from build123d import *

# Parameters (mm, degrees)
F0_W     = 21
F0_H     = 21
F1_DEPTH = 11
F3_DEPTH = 21.001
F5_DEPTH = 25
F6_W     = 0.76
F6_H     = 0.76
F7_DEPTH = 5.8


with BuildPart() as f1:
    # F0 (on Top) → F1 (new body)
    with BuildSketch(Plane.XY):
        with Locations((10.5, 10.5)):
            Rectangle(F0_W, F0_H)
    extrude(amount=F1_DEPTH)

    # F2 (on face) → F3 (cut, through all)
    with BuildSketch(Plane.XZ):
        Polygon((0, 11), (0, 0), (0.6, 11), align=None)
        Polygon((20.4, 11), (21, 0), (21, 11), align=None)
    extrude(amount=-F3_DEPTH, mode=Mode.SUBTRACT)

    # F4 (on Right) → F5 (cut)
    with BuildSketch(Plane.YZ):
        Polygon((20.4, 11), (21, 0), (21, 11), align=None)
        Polygon((0, 11), (0, 0), (0.6, 11), align=None)
    extrude(amount=F5_DEPTH, mode=Mode.SUBTRACT)

    # F6 (on face) → F7 (join)
    with BuildSketch(Plane(origin=(0, 0, 0), x_dir=(1, 0, 0), z_dir=(0, 0, -1))):
        with Locations((2.5, -2.38)):
            Rectangle(F6_W, F6_H)
        with Locations((5, -2.38)):
            Rectangle(F6_W, F6_H)
        with Locations((7.5, -2.38)):
            Rectangle(F6_W, F6_H)
        with Locations((10, -2.38)):
            Rectangle(F6_W, F6_H)
        with Locations((12.5, -2.38)):
            Rectangle(F6_W, F6_H)
        with Locations((18.5, -2.38)):
            Rectangle(F6_W, F6_H)
    extrude(amount=F7_DEPTH)


solid = f1.part
Read the model definition and answer for the solid it produces. Units are mm, in the model's axes. Give positions to 0.01 mm unless a question says otherwise; leave off trailing zeros. Loops run counter-clockwise (first coordinate to the right, second up) from the corner with the lowest first, then second, coordinate; pieces in that order, holes last. Notation, with made-up numbers: (59.5, -34.5) - (77.5, -34.5) arc R18 ccw to (77.5, -8.5) - close; hole circle Ø9 at (-30, -21). An arc over 180 degrees is marked (long way). Answer as CSV lines item,"result". Start each with the question number.
1) Find section D-D (z = 2.5). Write down the section's boundary in (x, y), then the cut area to 3 significant figures.
2) Straight lines are drawn through the part: L1, parallel to Z at x = 3, y = 13.25; L2, parallel to Y at x = 5, z = -1.5; L3, parallel to Y at x = 19.5, z = 8.5. For each, find the intervals that lie inside material, in ascending order. Write a range as from..to.
3) Find section C-C (y = 17.75). Write down the section's boundary in (x, z).
4) Find section A-A (z = -3.25). Write down the section's boundary in (x, y).
5) Find section B-B (x = 12.5). Write down the section's boundary in (y, z), then the cut area to 3 significant figures.
6) Each of these flat-tipped pins is pushed along its axis until it touches: pin 1 Ø0.6 at (x, z) = (5, -4) entering from +Y; pin 2 Ø3 at (x, y) = (10, 16) entering from -Z; pin 3 Ø4 at (x, z) = (7.5, 5) entering from +Y. Where does it stop, or does it pass through?
Findings below:
1,outline,"(0.14, 0.14) - (20.86, 0.14) - (20.86, 20.86) - (0.14, 20.86) - close"
1,area,"430 mm^2"
2,L1,"0..11"
2,L2,"2..2.76"
2,L3,"0.46..20.54"
3,outline,"(0, 0) - (21, 0) - (20.4, 11) - (0.6, 11) - close"
4,outline,"(2.12, 2) - (2.88, 2) - (2.88, 2.76) - (2.12, 2.76) - close; (4.62, 2) - (5.38, 2) - (5.38, 2.76) - (4.62, 2.76) - close; (7.12, 2) - (7.88, 2) - (7.88, 2.76) - (7.12, 2.76) - close; (9.62, 2) - (10.38, 2) - (10.38, 2.76) - (9.62, 2.76) - close; (12.12, 2) - (12.88, 2) - (12.88, 2.76) - (12.12, 2.76) - close; (18.12, 2) - (18.88, 2) - (18.88, 2.76) - (18.12, 2.76) - close"
5,outline,"(0, 0) - (2, 0) - (2, -5.8) - (2.76, -5.8) - (2.76, 0) - (21, 0) - (20.4, 11) - (0.6, 11) - close"
5,area,"229 mm^2"
6,pin 1,"y = 2.76"
6,pin 2,"z = 0"
6,pin 3,"y = 20.84"
